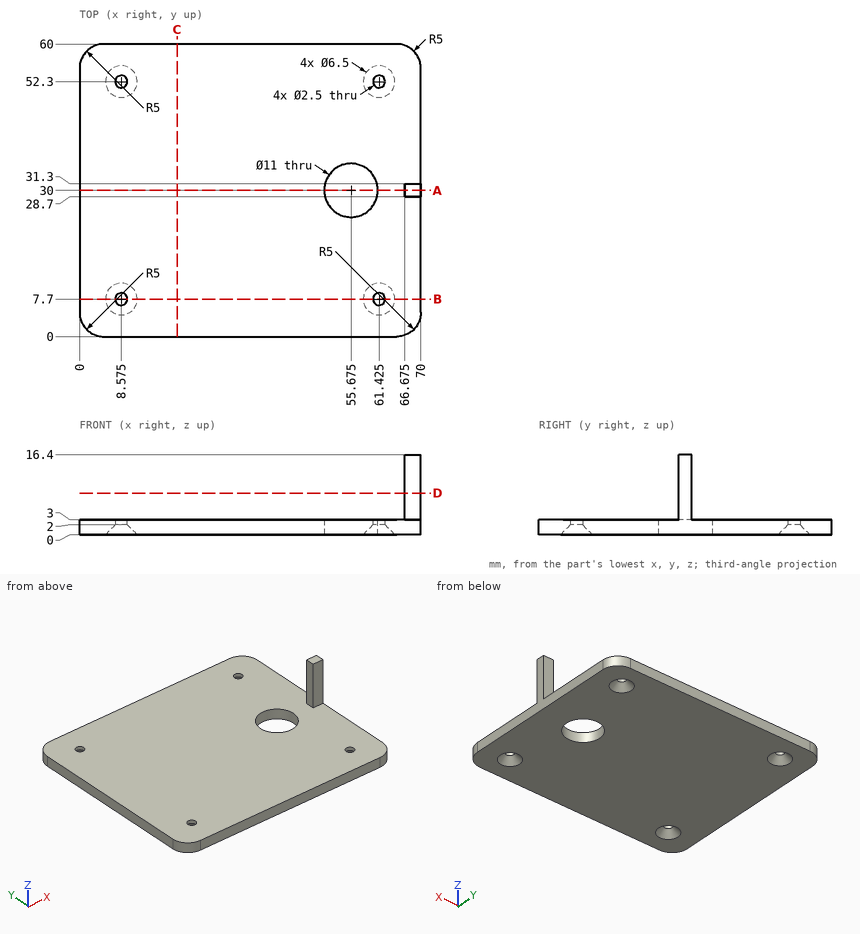
The figure shows three views and two pictorial views of one solid part (mm, origin at its lowest corner). Answer the questions. Coordinates: 2 decimals unless noted, no trailing zeros. Loops run counter-clockwise (first coordinate to the right, second up) from the corner with the lowest first, then second, coordinate; pieces in that order, holes last. Notation, with made-up numbers: M 66.25,82 L 87.25,82 A10 cw 87.25,91 Z; hole C 57.25,-22 d1. An arc over 180 degrees is marked long. Answer as CSV lines item,"result". Start each with the question number.
(1) The part is cut by section B-B (y = 7.7). Give the vertices of the cut face in (x, z) (3 decimals), and give its area (3 significant figures).
(2) The part is cut by section D-D (z = 8.5). Give the vertices of the cut face in (x, y) (3 decimals).
(3) The part is cut by section C-C (x = 20). Give the vertices of the cut face in (y, z), and give its area (3 significant figures).
(4) The part is cut by section A-A (y = 30). Give the vertices of the cut face in (x, z) (3 decimals).
(5) Given pin 1 (3 mm diameter, centred on x = 8.575, y = 7.7, fed in from +Z); pin 2 (2 mm diameter, centred on x = 8.575, y = 52.3, fed in from -Z); pin 3 (3 mm diameter, centred on x = 61.425, y = 7.7, fed in from -Z); pin 4 (3 mm diameter, centred on y = 30, z = 12, fed in from -X) (3 decimals), each flat-ended and moving along its own axis, determine where each tip first touches the part or whether it passes through.
(6) Find the intervals of material crossed by L1, parallel to X at y = 52.3, z = 2.4 (3 decimals); L2, parallel to Z at x = 26.5, y = 30.5; L3, parallel to Y at x = 57.5, z = 1, in increasing order. Write a range as [from, to].
Determined:
1,outline,"M 0,0 L 5.325,0 L 7.325,2 L 7.325,3 L 0,3 Z; M 9.825,2 L 11.825,0 L 58.175,0 L 60.175,2 L 60.175,3 L 9.825,3 Z; M 62.675,2 L 64.675,0 L 70,0 L 70,3 L 62.675,3 Z"
1,area,"187 mm2"
2,outline,"M 66.675,28.7 L 70,28.7 L 70,31.3 L 66.675,31.3 Z"
3,outline,"M 0,0 L 60,0 L 60,3 L 0,3 Z"
3,area,"180 mm2"
4,outline,"M 0,0 L 50.175,0 L 50.175,3 L 0,3 Z; M 61.175,0 L 70,0 L 70,16.4 L 66.675,16.4 L 66.675,3 L 61.175,3 Z"
5,pin 1,"z = 3"
5,pin 2,"through"
5,pin 3,"z = 1.75"
5,pin 4,"x = 66.675"
6,L1,"[0, 7.325], [9.825, 60.175], [62.675, 70]"
6,L2,"[0, 3]"
6,L3,"[0, 24.81], [35.19, 60]"
